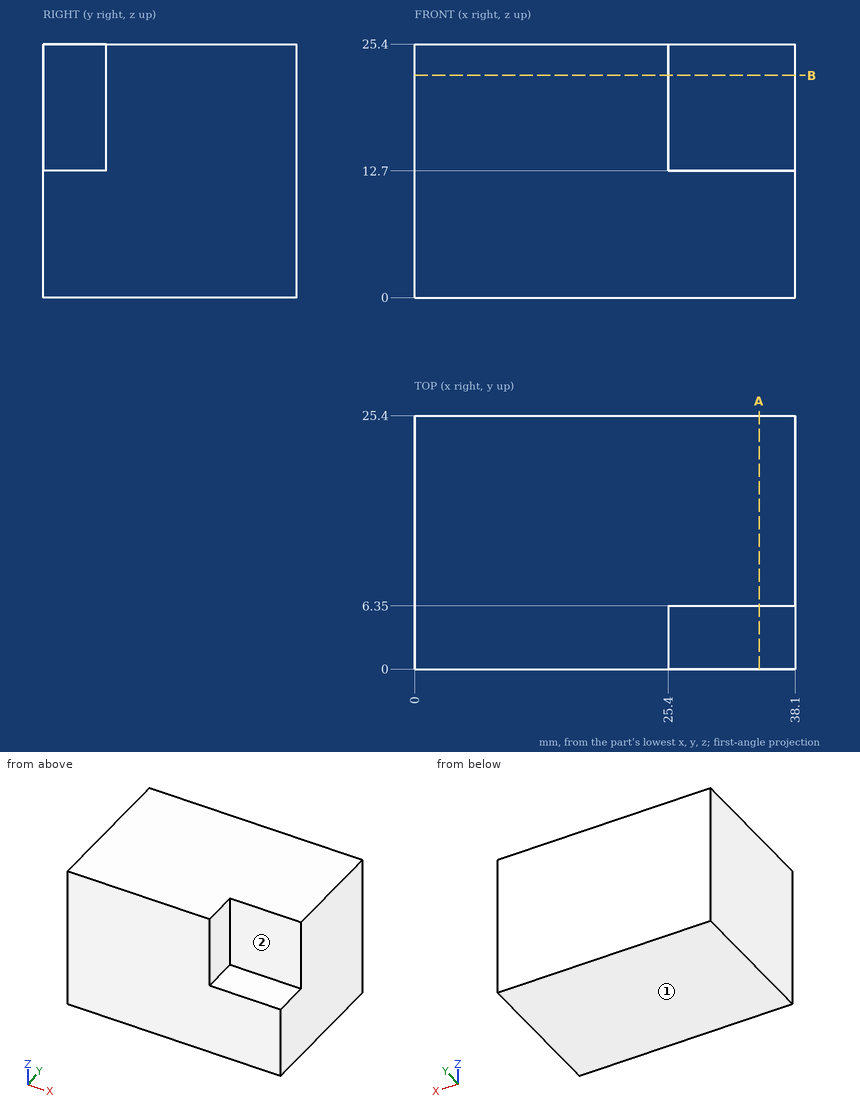
Here's the drawing with two shaded views (mm, measured from the low corner). I have some questions. A direction names the side the tool comes from. Round coordinates to 2 decimals unless told otherwise and drop trailing zeros. Loops run counter-clockwise (first coordinate to the right, second up) from the corner with the lowest first, then second, coordinate; pieces in that order, holes last.
1. Suppose I cut it at A-A, the plane x = 34.5. Please give me the cut outline in (y, z).
Answers:
outline: (0, 0) - (25.4, 0) - (25.4, 25.4) - (6.35, 25.4) - (6.35, 12.7) - (0, 12.7) - close
2. Will these pins go through, and if not, where does the flat tip stop? pin 1 (6.5 mm diameter, centred on x = 34.5, z = 16.5, fed in from -Y); pin 2 (1.9 mm diameter, centred on y = 2.5, z = 21.5, fed in from +X); pin 3 (3 mm diameter, centred on x = 33, y = 3.5, fed in from +Z).
Answers:
pin 1: stops at y = 6.35
pin 2: stops at x = 25.4
pin 3: stops at z = 12.7
3. If I drill on probe 1 along Y at (x, z) = (34, 17.5); probe 2 along X at (y, z) = (3, 13.75), over which ranges is the centre line in solid material (lowest first)?
Answers:
probe 1: y = 6.35 to 25.4
probe 2: x = 0 to 25.4
4. For the marked faces 1 and 2, which set-ups out of +Z, -Z, +X, -X, +Y, -Y let a thin tool reach every point of the face, with its end or its side?
Answers:
face 1: -Z, +X, -X, +Y, -Y
face 2: +Z, +X, -Y
5. Suppose I cut it at B-B, the plane z = 22.25. Please give me the cut outline in (x, y), and give its area (3 significant figures).
Answers:
outline: (0, 0) - (25.4, 0) - (25.4, 6.35) - (38.1, 6.35) - (38.1, 25.4) - (0, 25.4) - close
area: 887 mm2
